Here's how the part is built. I have some questions about the finished solid (model axes, mm). Coordinates: 2 decimals unless noted, no trailing zeros. Write each loop counter-clockwise with the first axis right and the second up, starting at its lowest first coordinate (ties: lowest second). Pieces come first, ordered by that corner, then holes. Notation, with made-up numbers: M 79.5,43 L 111.5,43 A23 ccw 111.5,79 Z; hole C 23,78.25 d3. An arc over 180 degrees is marked long. Write each question's results on one line, items separated by ' | '. Start each with the question number.
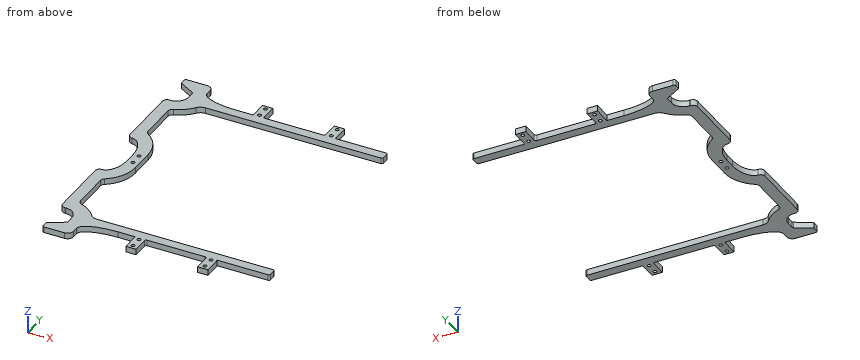
from build123d import *

# Parameters (mm, degrees)
SKETCH_1_R          = 1.5
SKETCH_1_W          = 10
SKETCH_1_H          = 20
EXTRUDE_1_DEPTH     = 5
FILLET_1_R          = 1.5
FILLET_2_R          = 8
EXTRUDE_5_DEPTH     = 5
SKETCH_7_R          = 1.5
CUT_EXTRUDE_1_DEPTH = 259.028370533
FILLET_5_R          = 1.5
EXTRUDE_6_DEPTH     = 5
SKETCH_9_W          = 10
SKETCH_9_H          = 40
CUT_EXTRUDE_2_DEPTH = 259.028370533
FILLET_6_R          = 4
FILLET_8_R          = 10
FILLET_9_R          = 10
FILLET_10_DEPTH     = 5
FILLET_11_DEPTH     = 5
FILLET_13_SIZE      = 10
FILLET_13_SIZE_2    = 30
FILLET_14_SIZE      = 30
FILLET_14_SIZE_2    = 10
FILLET_15_R         = 5
FILLET_16_R         = 30
FILLET_17_R         = 30
FILLET_18_R         = 30


with BuildPart() as part:
    # 草图1 → 凸台-拉伸1 (new body)
    # profile 1 of 3: a face of its own
    with BuildSketch(Plane.XY):
        Polygon((105.75, 0), (114.65, 0), (159.2, 0), (159.2, -8), (114.55, -8), (114.55, -23), (105.75, -23), (105.75, -8), (53.35, -8), (53.35, -23), (44.55, -23), (44.55, -8), (-10, -8), (-10, 183), (44.55, 183), (44.55, 198), (53.35, 198), (53.35, 183), (105.75, 183), (105.75, 198), (114.55, 198), (114.55, 183), (159.2, 183), (159.2, 175), (114.65, 175), (105.75, 175), (53.35, 175), (44.55, 175), (0, 175), (0, 0), (44.55, 0), (53.35, 0), align=None)
        with Locations((48.95, -10)):
            Circle(SKETCH_1_R, mode=Mode.SUBTRACT)
        with Locations((110.15, -19.5)):
            Circle(SKETCH_1_R, mode=Mode.SUBTRACT)
        with Locations((110.15, -10)):
            Circle(SKETCH_1_R, mode=Mode.SUBTRACT)
        with Locations((110.15, 194.5)):
            Circle(SKETCH_1_R, mode=Mode.SUBTRACT)
        with Locations((48.95, 194.5)):
            Circle(SKETCH_1_R, mode=Mode.SUBTRACT)
        with Locations((48.95, 185)):
            Circle(SKETCH_1_R, mode=Mode.SUBTRACT)
        with Locations((110.15, 185)):
            Circle(SKETCH_1_R, mode=Mode.SUBTRACT)
        with Locations((48.95, -19.5)):
            Circle(SKETCH_1_R, mode=Mode.SUBTRACT)
    # profile 2 of 3: a face of its own
    with BuildSketch(Plane.XY):
        with Locations((-5, 193)):
            Rectangle(SKETCH_1_W, SKETCH_1_H)
    # profile 3 of 3: a face of its own
    with BuildSketch(Plane.XY):
        with Locations((-5, -18)):
            Rectangle(SKETCH_1_W, SKETCH_1_H)
    extrude(amount=EXTRUDE_1_DEPTH)

    # 圆角1
    fillet_1_edges = [part.edges().sort_by_distance(p)[0] for p in [
        (159.2, 0, 2.5),
        (159.2, -8, 2.5),
        (105.75, -8, 2.5),
        (53.35, -8, 2.5),
        (53.35, 183, 2.5),
        (105.75, 183, 2.5),
        (159.2, 183, 2.5),
        (159.2, 175, 2.5),
    ]]
    fillet(fillet_1_edges, radius=FILLET_1_R)

    # 圆角2
    fillet_2_edges = [part.edges().sort_by_distance(p)[0] for p in [
        (0, 175, 2.5),
        (0, 0, 2.5),
    ]]
    fillet(fillet_2_edges, radius=FILLET_2_R)

    # 草图6 → 凸台-拉伸5 (add)
    with BuildSketch(Plane.XY.offset(5)):
        Polygon((-24, 197), (-10, 188.917096231), (-10, 203), (-24, 203), align=None)
        Polygon((-10, -28), (-24, -28), (-24, -22), (-10, -13.917096231), align=None)
    extrude(amount=-EXTRUDE_5_DEPTH)

    # 草图7 → 切除-拉伸1 (cut, through all)
    with BuildSketch(Plane(origin=(0, 0, 5), x_dir=(-1, 0, 0), z_dir=(0, 0, -1))):
        with Locations((5, 92.5)):
            Circle(SKETCH_7_R)
        with Locations((5, 82.5)):
            Circle(SKETCH_7_R)
    extrude(amount=CUT_EXTRUDE_1_DEPTH, mode=Mode.SUBTRACT)

    # 圆角5
    fillet_5_edges = [part.edges().sort_by_distance(p)[0] for p in [
        (-24, 203, 2.5),
        (-10, 188.917096231, 2.5),
        (-10, -13.917096231, 2.5),
        (-24, -28, 2.5),
    ]]
    fillet(fillet_5_edges, radius=FILLET_5_R)

    # 草图8 → 凸台-拉伸6 (add, through all)
    with BuildSketch(Plane(origin=(0, 0, 0), x_dir=(-1, 0, 0), z_dir=(0, 0, -1))):
        Polygon((25, 112), (10, 112), (10, 122), (15, 122), (15, 162), (10, 162), (10, 172), (25, 172), align=None)
        Polygon((15, 53), (10, 53), (10, 63), (25, 63), (25, 3), (10, 3), (10, 13), (15, 13), align=None)
    extrude(amount=-EXTRUDE_6_DEPTH)

    # 草图9 → 切除-拉伸2 (cut, through all)
    with BuildSketch(Plane(origin=(0, 0, 0), x_dir=(-1, 0, 0), z_dir=(0, 0, -1))):
        with Locations((5, 142)):
            Rectangle(SKETCH_9_W, SKETCH_9_H)
        with Locations((5, 33)):
            Rectangle(SKETCH_9_W, SKETCH_9_H)
    extrude(amount=-CUT_EXTRUDE_2_DEPTH, mode=Mode.SUBTRACT)

    # 圆角6
    fillet_6_edges = [part.edges().sort_by_distance(p)[0] for p in [
        (-25, 172, 2.5),
        (-25, 112, 2.5),
        (-15, 122, 2.5),
        (-15, 162, 2.5),
        (-25, 63, 2.5),
        (-25, 3, 2.5),
        (-15, 13, 2.5),
        (-15, 53, 2.5),
    ]]
    fillet(fillet_6_edges, radius=FILLET_6_R)

    # 圆角8
    fillet_8_edges = [part.edges().sort_by_distance(p)[0] for p in [
        (-10, 172, 2.5),
    ]]
    fillet(fillet_8_edges, radius=FILLET_8_R)

    # 圆角9
    fillet_9_edges = [part.edges().sort_by_distance(p)[0] for p in [
        (-10, 3, 2.5),
    ]]
    fillet(fillet_9_edges, radius=FILLET_9_R)

    # 圆角10: read off the stored shape, not the designer's step
    # 圆角10 outline → 圆角10 (add)
    with BuildSketch(Plane.XY):
        with BuildLine():
            Line((-10, 63), (-10, 82.979157617))
            add(Edge.make_bspline(
                [(-10, 82.979157617), (-10, 63.462208461), (-21.166666667, 62.996526269)],
                knots=[0, 0, 0, 1, 1, 1], degree=2, weights=[1, 0.721687836, 1]))
            ThreePointArc((-21.166666667, 62.996526269), (-21.083351432, 62.999131473), (-21, 63))
            Line((-21, 63), (-10, 63))
        make_face()
    extrude(amount=FILLET_10_DEPTH)

    # 圆角11: read off the stored shape, not the designer's step
    # 圆角11 outline → 圆角11 (add)
    with BuildSketch(Plane.XY):
        with BuildLine():
            ThreePointArc((-21, 112), (-21.083351432, 112.000868527), (-21.166666667, 112.003473731))
            add(Edge.make_bspline(
                [(-21.166666667, 112.003473731), (-10, 111.537791539), (-10, 92.020842383)],
                knots=[0, 0, 0, 1, 1, 1], degree=2, weights=[1, 0.721687836, 1]))
            Line((-10, 92.020842383), (-10, 112))
            Line((-10, 112), (-21, 112))
        make_face()
    extrude(amount=FILLET_11_DEPTH)

    # 圆角13
    # a fillet whose section is not a circle: 30, 10 mm, written as the material it adds along each edge
    with BuildSketch(Plane(origin=(0, 183, 0), x_dir=(0, 1, 0), z_dir=(0, 0, 1))) as fillet_13_piece_1:
        with BuildLine():
            Bezier((FILLET_13_SIZE, 0), (0, 0), (0, -FILLET_13_SIZE_2), weights=[1, 0.707106781, 1])
            Line((0, -FILLET_13_SIZE_2), (0, 0))
            Line((0, 0), (FILLET_13_SIZE, 0))
        make_face()
    extrude(amount=5)

    # 圆角14
    # a fillet whose section is not a circle: 30, 10 mm, written as the material it adds along each edge
    with BuildSketch(Plane(origin=(0, -8, 0), x_dir=(1, 0, 0), z_dir=(0, 0, 1))) as fillet_14_piece_1:
        with BuildLine():
            Bezier((FILLET_14_SIZE, 0), (0, 0), (0, -FILLET_14_SIZE_2), weights=[1, 0.707106781, 1])
            Line((0, -FILLET_14_SIZE_2), (0, 0))
            Line((0, 0), (FILLET_14_SIZE, 0))
        make_face()
    extrude(amount=5)

    # 圆角15
    fillet_15_edges = [part.edges().sort_by_distance(p)[0] for p in [
        (0, -28, 2.5),
        (0, 203, 2.5),
    ]]
    fillet(fillet_15_edges, radius=FILLET_15_R)

    # 圆角16
    fillet_16_edges = [part.edges().sort_by_distance(p)[0] for p in [
        (0, 162, 2.5),
    ]]
    fillet(fillet_16_edges, radius=FILLET_16_R)

    # 圆角17
    fillet_17_edges = [part.edges().sort_by_distance(p)[0] for p in [
        (0, 13, 2.5),
    ]]
    fillet(fillet_17_edges, radius=FILLET_17_R)

    # 圆角18
    fillet_18_edges = [part.edges().sort_by_distance(p)[0] for p in [
        (0, 53, 2.5),
        (0, 122, 2.5),
    ]]
    fillet(fillet_18_edges, radius=FILLET_18_R)


solid = part.part
1) I want a section at B-B, the plane z = 4.05. Give the number of separate pieces and of enclosed holes in the cut face, then the cut area to 3 significant figures.
2) For pin 1 Ø1.5 at (x, z) = (145, 3.5) entering from -Y; pin 2 Ø2.5 at (x, y) = (-5, 92.5) entering from +Z; pin 3 Ø1 at (y, z) = (68.5, 3) entering from +X; pin 4 Ø1.5 at (y, z) = (185, 2.5) entering from -X, each with a flat end and sliding along its axis, tell me the tip position at first contact or that it passes through.
3) Please list where these lines run through material, in increasing order: line 1 (Y direction, x = 149.5, z = 1.7); line 2 (Y direction, x = 48.95, z = 2.8); line 3 (Y direction, x = -4, z = 0.75). Write a range as [from, to].
4) I want a section at A-A, the plane x = 73. Write out the boundary of the cut face in (y, z), then the cut area to 3 significant figures.
5) I want a section at C-C, the plane y = 38.5. Write out the boundary of the cut face in (x, z).
Output:
1) separate pieces: 1 | enclosed holes: 10 | area: 6,220 mm2
2) pin 1: stops at y = -8 | pin 2: passes through | pin 3: stops at x = -1.14 | pin 4: stops at x = -10
3) line 1: y = [-8, 0], [175, 183] | line 2: y = [-23, -21], [-18, -11.5], [-8.5, 0], [175, 183.5], [186.5, 193], [196, 198] | line 3: y = [-27.9, 8.76], [62.23, 81.38], [83.62, 91.38], [93.62, 112.77], [166.24, 202.9]
4) outline: M -8,0 L 0,0 L 0,5 L -8,5 Z; M 175,0 L 183,0 L 183,5 L 175,5 Z | area: 80.0 mm2
5) outline: M -25,0 L -15,0 L -15,5 L -25,5 Z
